from build123d import *

# Parameters (mm, degrees)
SKETCH_1_R               = 102.5
SM_BASE_FLANGE_1_DEPTH   = 1
HOLE_WIZARD_8_0_8_1_D    = 8
PATTERN_CIRCULAR_1_COUNT = 6
HOLE_WIZARD_3_3_3_3_1_D  = 3.3


# Sheet-metal steps are written as plain solids
with BuildPart() as part:
    # Sketch 1 → 基体-法兰1 (new body)
    with BuildSketch(Plane(origin=(0, 0, 0), x_dir=(1, 0, 0), z_dir=(0, 1, 0))):
        with Locations(Location((0, 0, 0), (0, 0, 270))):
            Circle(SKETCH_1_R)
        Polygon((-12.990381057, 37.5), (0, 60), (12.990381057, 37.5), (0, 45), align=None, mode=Mode.SUBTRACT)
        Polygon((30, 0), (15, 25.980762114), (-15, 25.980762114), (-30, 0), (-15, -25.980762114), (15, -25.980762114), align=None, mode=Mode.SUBTRACT)
    extrude(amount=-SM_BASE_FLANGE_1_DEPTH)

    # Ø8.0 (8) 直径孔1 (through all)
    with Locations(Plane(origin=(0, 0, 0), x_dir=(1, 0, 0), z_dir=(0, 1, 0))):
        with Locations((-90, 0)):
            hole_wizard_8_0_8_1 = Hole(HOLE_WIZARD_8_0_8_1_D / 2)

    # 阵列(圆周)1: Ø8.0 (8) 直径孔1 ×6 about axis
    pattern_circular_1_axis = Axis((0, 0, 0), (0, 1, 0))
    for i in range(1, PATTERN_CIRCULAR_1_COUNT):
        add(hole_wizard_8_0_8_1.rotate(pattern_circular_1_axis, i * 360 / PATTERN_CIRCULAR_1_COUNT), mode=Mode.SUBTRACT)

    # Ø3.3 (3.3) 直径孔1 (through all)
    with Locations(Plane(origin=(0, 0, 0), x_dir=(1, 0, 0), z_dir=(0, 1, 0))):
        with Locations((32.5, -56.291651246), (65, 0), (32.5, 56.291651246), (-32.5, 56.291651246), (-65, 0), (-32.5, -56.291651246)):
            Hole(HOLE_WIZARD_3_3_3_3_1_D / 2)


solid = part.part
Geometry check sheet. Reference: the model listing, model coordinates, mm. A direction names the side the tool comes from. Give positions to 0.01 mm unless a question says otherwise; leave off trailing zeros. Loops run counter-clockwise (first coordinate to the right, second up) from the corner with the lowest first, then second, coordinate; pieces in that order, holes last. Notation, with made-up numbers: M 29.25,72.5 L 53.25,72.5 A28 ccw 53.25,109.5 Z; hole C 29,24.5 d11. An arc over 180 degrees is marked long. Write each question's results on one line, items separated by ' | '.
1) Tool access check on faces 1 (the face through (-21, 0, 21)), 2 (the face through (-22.395, -0.493, -13.172)). Record the directions out of +Z, -Z, +X, -X, +Y, -Y that give a thin tool (end or side, any length) a straight path to the whole face; none if there is none.
Answers follow:
face 1: +Z, -Z, +X, -X, +Y | face 2: +Y, -Y
2) Section check A-A, the plane x = -90. Record the boundary of the cut face in (y, z), plus the area to 3 significant figures.
Answers follow:
outline: M -1,-49.05 L 0,-49.05 L 0,-4 L -1,-4 Z; M -1,4 L 0,4 L 0,49.05 L -1,49.05 Z | area: 90.1 mm2
3) Section check C-C, the plane y = -0.4. Count the separate pieces of the cut face and the enclosed holes in it, plus the area to 3 significant figures.
Answers follow:
separate pieces: 1 | enclosed holes: 14 | area: 30,100 mm2
4) Gauge pin test, flat ends, axial feed: pin 1 (7 mm diameter, centred on x = -90, z = 0, fed in from -Y); pin 2 (13 mm diameter, centred on x = -45, z = -77.94, fed in from -Y). Record the tip position at first contact, or that the pin passes through.
Answers follow:
pin 1: through | pin 2: y = -1
5) Release check for a two-part mould opening along X. For faces 3 (the face through (-6.586, -0.493, -48.592)), 4 (the face through (-100.063, -0.493, -22.22)), 5 (the face through (-21, -1, 21)), 6 (the face through (22.605, -0.493, -12.809)) record: +X half, -X half, draft (parallel to the pull), parting line (faces both ways), or undercut.
Answers follow:
face 3: undercut | face 4: parting line | face 5: draft | face 6: undercut
6) Section check D-D, the plane z = -70.5. Record the boundary of the cut face in (x, y), plus the area to 3 significant figures.
Answers follow:
outline: M -74.4,-1 L 74.4,-1 L 74.4,0 L -74.4,0 Z | area: 149 mm2
7) Section check B-B, the plane z = 14.5. Record the boundary of the cut face in (x, y), plus the area to 3 significant figures.
Answers follow:
outline: M -101.47,-1 L -21.63,-1 L -21.63,0 L -101.47,0 Z; M 21.63,-1 L 101.47,-1 L 101.47,0 L 21.63,0 Z | area: 160 mm2
8) Thickness scan on line 1 (X direction, y = -0.1, z = 76); line 2 (Z direction, x = -45, y = -0.65); line 3 (Z direction, x = -5.5, y = -0.55). Record the ranges inside material, lowest first.
Answers follow:
line 1: -68.78 to -48.5, -41.5 to 41.5, 48.5 to 68.78 | line 2: -92.09 to -81.94, -73.94 to 73.94, 81.94 to 92.09 | line 3: -102.35 to -50.47, -41.82 to -25.98, 25.98 to 102.35
